The listing builds one solid part. Answer for the finished solid, in the listing's coordinates (mm). A direction names the side the tool comes from. Round coordinates to 2 decimals unless told otherwise and drop trailing zeros. Write each loop counter-clockwise with the first axis right and the second up, starting at its lowest first coordinate (ties: lowest second). Pieces come first, ordered by that corner, then holes.
(1) A cutting plane is placed at B-B, the plane y = 7. Give the number of separate pieces and of enclosed holes in the cut face, and give its area (3 significant figures).
(2) A cutting plane is placed at A-A, the plane z = 20. Give the vertices of the cut face in (x, y).
(3) Find the intervals of material crossed by probe 1 along Y at (x, z) = (20, -46); probe 2 along X at (y, z) = (34, 47); probe 3 along Z at (x, y) = (0, 40.85), in increasing order.
(4) Each of these flat-tipped pins is pushed along its axis until it touches: pin 1 Ø5 at (x, z) = (-26, 25.5) entering from +Y; pin 2 Ø8 at (x, y) = (1, 31.5) entering from -Z; pin 3 Ø12 at (x, y) = (0.5, 26.5) entering from -Z. Where does it stop, or does it pass through?
(5) The mould has two halves that part along X. Classify faces 5 (the face through (-36, 40, -40)), 6 (the face through (42.534, 20.734, 34.112)), 7 (the face through (52, 40, 12)), 8 (the face through (-10.58, 40.99, 47.64)): +X half, -X half, draft (parallel to the pull), parting line (faces both ways), or undercut.
(6) For faces 1 (the face through (-19.299, 20.734, 50.993)), 2 (the face through (2.596, 20.734, -54.461)), 3 (the face through (6, 40, 54)), 4 (the face through (-0.1, 12, 4.3)), determine the directions among +Z, -Z, +X, -X, +Y, -Y from which every point of the face is accessible in a straight line to the end or side of a thin tool.
from build123d import *

# Parameters (mm, degrees)
SKETCH2_R           = 59
BOSS_EXTRUDE1_DEPTH = 2
BOSS_EXTRUDE2_DEPTH = 38
SKETCH4_R           = 59
SKETCH4_R_2         = 48.802353881
BOSS_EXTRUDE3_DEPTH = 2
SKETCH5_R           = 10
SKETCH5_R_2         = 4
BOSS_EXTRUDE4_DEPTH = 10
SKETCH6_R           = 1.5
CUT_EXTRUDE1_DEPTH  = 25
SKETCH7_R           = 4
CUT_EXTRUDE2_DEPTH  = 3


with BuildPart() as part:
    # Sketch2 → Boss-Extrude1 (new body)
    with BuildSketch(Plane(origin=(0, 0, 0), x_dir=(1, 0, 0), z_dir=(0, 1, 0))):
        Circle(SKETCH2_R)
    extrude(amount=BOSS_EXTRUDE1_DEPTH)

    # Sketch3 → Boss-Extrude2 (add)
    with BuildSketch(Plane(origin=(0, 2, 0), x_dir=(1, 0, 0), z_dir=(0, 1, 0))):
        with BuildLine():
            Line((-14.892857143, 46.474428995), (-14, 48.26406754))
            ThreePointArc((-14, 48.26406754), (-12.934313455, 53.621635593), (-9.899494937, 58.163562477))
            ThreePointArc((-9.899494937, 58.163562477), (-10.714001991, 58.019049986), (-11.526402854, 57.863131934))
            ThreePointArc((-11.526402854, 57.863131934), (-14.384712835, 52.516130174), (-14.892857143, 46.474428995))
        make_face()
        with BuildLine():
            Line((0.197439531, 48.801954489), (1.599625859, 50.228093858))
            ThreePointArc((1.599625859, 50.228093858), (4.268733569, 54.994128614), (8.558550091, 58.375947276))
            ThreePointArc((8.558550091, 58.375947276), (7.739251034, 58.490204252), (6.918430571, 58.592963045))
            ThreePointArc((6.918430571, 58.592963045), (2.547701825, 54.390928538), (0.197439531, 48.801954489))
        make_face()
        with BuildLine():
            Line((15.268409449, 46.352404654), (17.042669195, 47.27544439))
            ThreePointArc((17.042669195, 47.27544439), (21.05392721, 50.983413159), (26.178824605, 52.874087626))
            ThreePointArc((26.178824605, 52.874087626), (25.434932246, 53.2359298), (24.686039809, 53.587306692))
            ThreePointArc((24.686039809, 53.587306692), (19.230729681, 50.941563853), (15.268409449, 46.352404654))
        make_face()
        with BuildLine():
            Line((28.844801068, 39.365558495), (30.817457326, 39.695145037))
            ThreePointArc((30.817457326, 39.695145037), (35.778215764, 41.982086001), (41.236533368, 42.196543884))
            ThreePointArc((41.236533368, 42.196543884), (40.640865073, 42.770551623), (40.037207473, 43.336151396))
            ThreePointArc((40.037207473, 43.336151396), (34.031319726, 42.505683967), (28.844801068, 39.365558495))
        make_face()
        with BuildLine():
            Line((39.597662585, 28.525337195), (41.575618016, 28.229208316))
            ThreePointArc((41.575618016, 28.229208316), (47.000283277, 28.87125976), (52.257722933, 27.388508426))
            ThreePointArc((52.257722933, 27.388508426), (51.868586866, 28.118493853), (51.469254313, 28.842951659))
            ThreePointArc((51.469254313, 28.842951659), (45.500687087, 29.90905158), (39.597662585, 28.525337195))
        make_face()
        with BuildLine():
            Line((46.474428995, 14.892857143), (48.26406754, 14))
            ThreePointArc((48.26406754, 14), (53.621635593, 12.934313455), (58.163562477, 9.899494937))
            ThreePointArc((58.163562477, 9.899494937), (58.019049986, 10.714001991), (57.863131934, 11.526402854))
            ThreePointArc((57.863131934, 11.526402854), (52.516130174, 14.384712835), (46.474428995, 14.892857143))
        make_face()
        with BuildLine():
            Line((48.801954489, -0.197439531), (50.228093858, -1.599625859))
            ThreePointArc((50.228093858, -1.599625859), (54.994128614, -4.268733569), (58.375947276, -8.558550091))
            ThreePointArc((58.375947276, -8.558550091), (58.490204252, -7.739251034), (58.592963045, -6.918430571))
            ThreePointArc((58.592963045, -6.918430571), (54.390928538, -2.547701825), (48.801954489, -0.197439531))
        make_face()
        with BuildLine():
            Line((46.352404654, -15.268409449), (47.27544439, -17.042669195))
            ThreePointArc((47.27544439, -17.042669195), (50.983413159, -21.05392721), (52.874087626, -26.178824605))
            ThreePointArc((52.874087626, -26.178824605), (53.2359298, -25.434932246), (53.587306692, -24.686039809))
            ThreePointArc((53.587306692, -24.686039809), (50.941563853, -19.230729681), (46.352404654, -15.268409449))
        make_face()
        with BuildLine():
            Line((39.365558495, -28.844801068), (39.695145037, -30.817457326))
            ThreePointArc((39.695145037, -30.817457326), (41.982086001, -35.778215764), (42.196543884, -41.236533368))
            ThreePointArc((42.196543884, -41.236533368), (42.770551623, -40.640865073), (43.336151396, -40.037207473))
            ThreePointArc((43.336151396, -40.037207473), (42.505683967, -34.031319726), (39.365558495, -28.844801068))
        make_face()
        with BuildLine():
            Line((28.525337195, -39.597662585), (28.229208316, -41.575618016))
            ThreePointArc((28.229208316, -41.575618016), (28.87125976, -47.000283277), (27.388508426, -52.257722933))
            ThreePointArc((27.388508426, -52.257722933), (28.118493853, -51.868586866), (28.842951659, -51.469254313))
            ThreePointArc((28.842951659, -51.469254313), (29.90905158, -45.500687087), (28.525337195, -39.597662585))
        make_face()
        with BuildLine():
            Line((14.892857143, -46.474428995), (14, -48.26406754))
            ThreePointArc((14, -48.26406754), (12.934313455, -53.621635593), (9.899494937, -58.163562477))
            ThreePointArc((9.899494937, -58.163562477), (10.714001991, -58.019049986), (11.526402854, -57.863131934))
            ThreePointArc((11.526402854, -57.863131934), (14.384712835, -52.516130174), (14.892857143, -46.474428995))
        make_face()
        with BuildLine():
            Line((-0.197439531, -48.801954489), (-1.599625859, -50.228093858))
            ThreePointArc((-1.599625859, -50.228093858), (-4.268733569, -54.994128614), (-8.558550091, -58.375947276))
            ThreePointArc((-8.558550091, -58.375947276), (-7.739251034, -58.490204252), (-6.918430571, -58.592963045))
            ThreePointArc((-6.918430571, -58.592963045), (-2.547701825, -54.390928538), (-0.197439531, -48.801954489))
        make_face()
        with BuildLine():
            Line((-15.268409449, -46.352404654), (-17.042669195, -47.27544439))
            ThreePointArc((-17.042669195, -47.27544439), (-21.05392721, -50.983413159), (-26.178824605, -52.874087626))
            ThreePointArc((-26.178824605, -52.874087626), (-25.434932246, -53.2359298), (-24.686039809, -53.587306692))
            ThreePointArc((-24.686039809, -53.587306692), (-19.230729681, -50.941563853), (-15.268409449, -46.352404654))
        make_face()
        with BuildLine():
            Line((-28.844801068, -39.365558495), (-30.817457326, -39.695145037))
            ThreePointArc((-30.817457326, -39.695145037), (-35.778215764, -41.982086001), (-41.236533368, -42.196543884))
            ThreePointArc((-41.236533368, -42.196543884), (-40.640865073, -42.770551623), (-40.037207473, -43.336151396))
            ThreePointArc((-40.037207473, -43.336151396), (-34.031319726, -42.505683967), (-28.844801068, -39.365558495))
        make_face()
        with BuildLine():
            Line((-39.597662585, -28.525337195), (-41.575618016, -28.229208316))
            ThreePointArc((-41.575618016, -28.229208316), (-47.000283277, -28.87125976), (-52.257722933, -27.388508426))
            ThreePointArc((-52.257722933, -27.388508426), (-51.868586866, -28.118493853), (-51.469254313, -28.842951659))
            ThreePointArc((-51.469254313, -28.842951659), (-45.500687087, -29.90905158), (-39.597662585, -28.525337195))
        make_face()
        with BuildLine():
            Line((-46.474428995, -14.892857143), (-48.26406754, -14))
            ThreePointArc((-48.26406754, -14), (-53.621635593, -12.934313455), (-58.163562477, -9.899494937))
            ThreePointArc((-58.163562477, -9.899494937), (-58.019049986, -10.714001991), (-57.863131934, -11.526402854))
            ThreePointArc((-57.863131934, -11.526402854), (-52.516130174, -14.384712835), (-46.474428995, -14.892857143))
        make_face()
        with BuildLine():
            Line((-48.801954489, 0.197439531), (-50.228093858, 1.599625859))
            ThreePointArc((-50.228093858, 1.599625859), (-54.994128614, 4.268733569), (-58.375947276, 8.558550091))
            ThreePointArc((-58.375947276, 8.558550091), (-58.490204252, 7.739251034), (-58.592963045, 6.918430571))
            ThreePointArc((-58.592963045, 6.918430571), (-54.390928538, 2.547701825), (-48.801954489, 0.197439531))
        make_face()
        with BuildLine():
            Line((-46.352404654, 15.268409449), (-47.27544439, 17.042669195))
            ThreePointArc((-47.27544439, 17.042669195), (-50.983413159, 21.05392721), (-52.874087626, 26.178824605))
            ThreePointArc((-52.874087626, 26.178824605), (-53.2359298, 25.434932246), (-53.587306692, 24.686039809))
            ThreePointArc((-53.587306692, 24.686039809), (-50.941563853, 19.230729681), (-46.352404654, 15.268409449))
        make_face()
        with BuildLine():
            Line((-39.365558495, 28.844801068), (-39.695145037, 30.817457326))
            ThreePointArc((-39.695145037, 30.817457326), (-41.982086001, 35.778215764), (-42.196543884, 41.236533368))
            ThreePointArc((-42.196543884, 41.236533368), (-42.770551623, 40.640865073), (-43.336151396, 40.037207473))
            ThreePointArc((-43.336151396, 40.037207473), (-42.505683967, 34.031319726), (-39.365558495, 28.844801068))
        make_face()
        with BuildLine():
            Line((-28.525337195, 39.597662585), (-28.229208316, 41.575618016))
            ThreePointArc((-28.229208316, 41.575618016), (-28.87125976, 47.000283277), (-27.388508426, 52.257722933))
            ThreePointArc((-27.388508426, 52.257722933), (-28.118493853, 51.868586866), (-28.842951659, 51.469254313))
            ThreePointArc((-28.842951659, 51.469254313), (-29.90905158, 45.500687087), (-28.525337195, 39.597662585))
        make_face()
    extrude(amount=BOSS_EXTRUDE2_DEPTH)

    # Sketch4 → Boss-Extrude3 (add)
    with BuildSketch(Plane(origin=(0, 40, 0), x_dir=(1, 0, 0), z_dir=(0, 1, 0))):
        Circle(SKETCH4_R)
        Circle(SKETCH4_R_2, mode=Mode.SUBTRACT)
    extrude(amount=BOSS_EXTRUDE3_DEPTH)

    # Sketch5 → Boss-Extrude4 (add)
    with BuildSketch(Plane(origin=(0, 2, 0), x_dir=(1, 0, 0), z_dir=(0, 1, 0))):
        Circle(SKETCH5_R)
        Circle(SKETCH5_R_2, mode=Mode.SUBTRACT)
    extrude(amount=BOSS_EXTRUDE4_DEPTH)

    # Sketch6 → Cut-Extrude1 (cut)
    with BuildSketch(Plane.XY):
        with Locations((0, 7)):
            Circle(SKETCH6_R)
    extrude(amount=-CUT_EXTRUDE1_DEPTH, mode=Mode.SUBTRACT)

    # Sketch7 → Cut-Extrude2 (cut, through all)
    with BuildSketch(Plane(origin=(0, 2, 0), x_dir=(1, 0, 0), z_dir=(0, 1, 0))):
        Circle(SKETCH7_R)
    extrude(amount=-CUT_EXTRUDE2_DEPTH, mode=Mode.SUBTRACT)


solid = part.part
Solutions:
1. separate pieces: 21
1. enclosed holes: 0
1. area: 478 mm2
2. outline: (-55.51, 0) - (55.51, 0) - (55.51, 2) - (51.49, 2) - (51.49, 40) - (55.51, 40) - (55.51, 42) - (44.52, 42) - (44.52, 40) - (50.27, 40) - (50.27, 2) - (-55.51, 2) - close; (-55.51, 40) - (-44.52, 40) - (-44.52, 42) - (-55.51, 42) - close
3. probe 1: y = 0 to 2, 40 to 42
3. probe 2: x = -16.51 to -15.65, 14.63 to 14.95, 28.87 to 29.87
3. probe 3: z = -59 to -48.8, 48.8 to 59
4. pin 1: stops at y = 2
4. pin 2: stops at z = -57.16
4. pin 3: stops at z = -58.32
5. face 5: undercut
5. face 6: +X half
5. face 7: draft
5. face 8: undercut
6. face 1: +Z
6. face 2: -Z
6. face 3: none
6. face 4: +Y
